Work out the finished part from the listing and answer in its coordinate system (mm). A direction names the side the tool comes from. Coordinates: 2 decimals unless noted, no trailing zeros. Write each loop counter-clockwise with the first axis right and the second up, starting at its lowest first coordinate (ties: lowest second). Pieces come first, ordered by that corner, then holes. Notation, with made-up numbers: (88, 28.5) -> (130, 28.5) arc R28 ccw to (130, 52.5) -> close; hole circle Ø11 at (13.25, 48). An arc over 180 degrees is marked (long way). Write each question's results on one line, items separated by ' | '. Start each with the question number.
from build123d import *

# Parameters (mm, degrees)
SKETCH_1_W          = 27.6
SKETCH_1_H          = 27.3
EXTRUDE_1_DEPTH     = 4
CUT_EXTRUDE_START   = 4
SKETCH_2_R          = 10
CUT_EXTRUDE_1_DEPTH = 0.3
SKETCH_2_3_R        = 6.921661
CUT_EXTRUDE_7_DEPTH = 0.6
SKETCH_2_5_R        = 1.127346788
SKETCH_2_5_R_2      = 3.020554036
CUT_EXTRUDE_8_DEPTH = 0.8
SKETCH_3_W          = 10
SKETCH_3_H          = 2
EXTRUDE_2_DEPTH     = 8


with BuildPart() as part:
    # 草图1 → 凸台-拉伸1 (new body)
    with BuildSketch(Plane.XY):
        Rectangle(SKETCH_1_W, SKETCH_1_H)
    extrude(amount=EXTRUDE_1_DEPTH)

    # 草图2 → 切除-拉伸1 (cut)
    with BuildSketch(Plane.XY.offset(CUT_EXTRUDE_START)):
        Circle(SKETCH_2_R)
    extrude(amount=-CUT_EXTRUDE_1_DEPTH, mode=Mode.SUBTRACT)

    # 草图2<3> → 切除-拉伸7 (cut)
    with BuildSketch(Plane.XY.offset(CUT_EXTRUDE_START)):
        Circle(SKETCH_2_3_R)
    extrude(amount=-CUT_EXTRUDE_7_DEPTH, mode=Mode.SUBTRACT)

    # 草图2<5> → 切除-拉伸8 (cut)
    with BuildSketch(Plane.XY.offset(CUT_EXTRUDE_START)):
        with Locations((-2.821175222, -4.128071022)):
            Circle(SKETCH_2_5_R)
        with Locations((3.223015918, 2.197908993)):
            Circle(SKETCH_2_5_R_2)
    extrude(amount=-CUT_EXTRUDE_8_DEPTH, mode=Mode.SUBTRACT)

    # 草图3 → 凸台-拉伸2 (add)
    with BuildSketch(Plane(origin=(0, 0, 0), x_dir=(-1, 0, 0), z_dir=(0, 0, -1))):
        with Locations((0, 12.65)):
            Rectangle(SKETCH_3_W, SKETCH_3_H)
    extrude(amount=EXTRUDE_2_DEPTH)


solid = part.part
1. Find section C-C on z = -2.25. Give the vertices of the cut face in (x, y), and give its area (3 significant figures).
2. For faces 1 (the face through (0, -13.65, 2)), 2 (the face through (5, 13, -4)), 3 (the face through (-5, 13, -4)), 4 (the face through (0, 0, 3.4)), determine the directions among +Z, -Z, +X, -X, +Y, -Y from which every point of the face is accessible in a straight line to the end or side of a thin tool.
3. Find section D-D on y = 12. Give the vertices of the cut face in (x, z).
4. Find the intervals of material crossed by L1, parallel to Y at x = 0, z = 3.65; L2, parallel to Z at x = -12, y = 12.5; L3, parallel to Y at x = 3.25, z = -1.25, in increasing order.
5. Find section B-B on x = -11.75. Give the vertices of the cut face in (y, z).
6. Given pin 1 Ø3.5 at (x, y) = (-2.82, -4.13) entering from +Z; pin 2 Ø3 at (x, z) = (10, -2.5) entering from -Y; pin 3 Ø3 at (x, y) = (-8.5, 7.5) entering from -Z; pin 4 Ø6.5 at (x, z) = (-1, -5.5) entering from -Y, each flat-ended and moving along its own axis, determine where each tip first touches the part or whether it passes through.
7. Determine the mould class of faces 5 (the face through (-3, -4, 3.2)), 6 (the face through (-2, -7, 3.7)), 7 (the face through (0, 11.65, -4)), 8 (the face through (0, 0, 0)) for opening direction Y: pulls with the +Y half, pulls with the -Y half, needs draft (parallel to the pull), parting line crosses it, or undercut.
Ans:
1) outline: (-5, 11.65) -> (5, 11.65) -> (5, 13.65) -> (-5, 13.65) -> close | area: 20.0 mm²
2) face 1: +Z, -Z, +X, -X, -Y | face 2: -Z, +X, +Y, -Y | face 3: -Z, -X, +Y, -Y | face 4: +Z
3) outline: (-13.8, 0) -> (-5, 0) -> (-5, -8) -> (5, -8) -> (5, 0) -> (13.8, 0) -> (13.8, 4) -> (-13.8, 4) -> close
4) L1: y = -13.65 to -6.92, 6.92 to 13.65 | L2: z = 0 to 4 | L3: y = 11.65 to 13.65
5) outline: (-13.65, 0) -> (13.65, 0) -> (13.65, 4) -> (-13.65, 4) -> close
6) pin 1: stops at z = 3.4 | pin 2: passes through | pin 3: stops at z = 0 | pin 4: stops at y = 11.65
7) face 5: undercut | face 6: undercut | face 7: pulls with the -Y half | face 8: needs draft
